Design review of the part built by this model. Coordinates are the model's own, in mm. Face numbers are marked on the shaded views. A direction names the side the tool comes from. Give positions to 0.01 mm unless a question says otherwise; leave off trailing zeros. Loops run counter-clockwise (first coordinate to the right, second up) from the corner with the lowest first, then second, coordinate; pieces in that order, holes last. Notation, with made-up numbers: M 62.5,27 L 76.5,27 A17 cw 76.5,55 Z; hole C 36,43.25 d4. An arc over 180 degrees is marked long. Use a Markdown table: item, result. Add a question column.
(1) Insertion check: pin 1 Ø10 at (x, z) = (-5, -10.5) entering from -Y; pin 2 Ø3 at (x, z) = (-13, 1) entering from +Y; pin 3 Ø0.9 at (x, y) = (32.5, -0.5) entering from -Z. Each pin has a flat end and moves straight along its axis. Give the tip position at first contact, or say it passes through.
(2) For probe 1 along Y at (x, z) = (0, 3.9); probe 2 along Y at (x, z) = (0, -8); probe 3 along X at (y, z) = (-32.5, -7.75), list the stretches that pass through material, from the lowest coordinate up.
(3) For the marked faces 1 and 2, list the 3-axis set-ups (+Z, -Z, +X, -X, +Y, -Y) from which the entire face can be reached by the end or side of a thin tool; tool diameter is ignored.
(4) Add section D-D, the plane z = 3.5. Give the boundary of the cut face in (x, y).
(5) Add section B-B, the plane y = -32.5. Give the boundary of the cut face in (x, z).
(6) Add section A-A, the plane z = -10.75. Give the boundary of the cut face in (x, y), then the cut area to 3 significant figures.
(7) Draft analysis for pull direction X (two halves, no side actions). For the marked faces 3 and 4, state which applies: pulls with the +X half, pulls with the -X half, needs draft (parallel to the pull), parting line crosses it, or undercut.
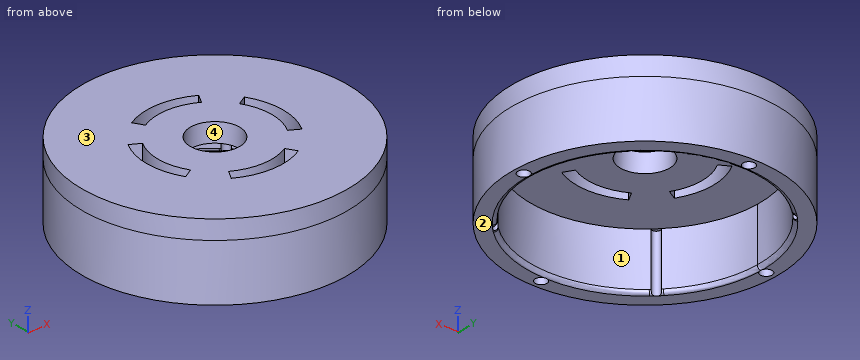
```python
from build123d import *

# Parameters (mm, degrees)
SKETCH_2_R          = 35
SKETCH_2_R_2        = 6.5
EXTRUDE_1_DEPTH     = 5
EXTRUDE_START       = 15
SKETCH_3_R          = 35
SKETCH_3_R_2        = 30.1
EXTRUDE_2_DEPTH     = 15
SKETCH_4_R          = 1.55
CUT_EXTRUDE_1_DEPTH = 10
CUT_EXTRUDE_2_DEPTH = 52.720402164
CUT_EXTRUDE_5_DEPTH = 15
FILLET_1_R          = 1


with BuildPart() as part:
    # 草图2 → 凸台-拉伸1 (new body)
    with BuildSketch(Plane.XY):
        Circle(SKETCH_2_R)
        Circle(SKETCH_2_R_2, mode=Mode.SUBTRACT)
    extrude(amount=EXTRUDE_1_DEPTH)

    # 草图3 → 凸台-拉伸2 (add)
    with BuildSketch(Plane(origin=(0, 0, 0), x_dir=(-1, 0, 0), z_dir=(0, 0, -1)).offset(EXTRUDE_START)):
        Circle(SKETCH_3_R)
        Circle(SKETCH_3_R_2, mode=Mode.SUBTRACT)
    extrude(amount=-EXTRUDE_2_DEPTH)

    # 草图4 → 切除-拉伸1 (cut)
    with BuildSketch(Plane(origin=(0, 0, -15), x_dir=(-1, 0, 0), z_dir=(0, 0, -1))):
        with Locations((0, 32.5)):
            Circle(SKETCH_4_R)
        with Locations((32.5, 0)):
            Circle(SKETCH_4_R)
        with Locations((0, -32.5)):
            Circle(SKETCH_4_R)
        with Locations((-32.5, 0)):
            Circle(SKETCH_4_R)
    extrude(amount=-CUT_EXTRUDE_1_DEPTH, mode=Mode.SUBTRACT)

    # 草图5 → 切除-拉伸2 (cut, through all)
    with BuildSketch(Plane(origin=(0, 0, 0), x_dir=(-1, 0, 0), z_dir=(0, 0, -1))):
        with BuildLine():
            Line((12.990381057, -7.5), (15.588457268, -9))
            ThreePointArc((15.588457268, -9), (18, 0), (15.588457268, 9))
            Line((15.588457268, 9), (12.990381057, 7.5))
            ThreePointArc((12.990381057, 7.5), (15, 0), (12.990381057, -7.5))
        make_face()
        with BuildLine():
            Line((-7.5, 12.990381057), (-9, 15.588457268))
            ThreePointArc((-9, 15.588457268), (0, 18), (9, 15.588457268))
            Line((9, 15.588457268), (7.5, 12.990381057))
            ThreePointArc((7.5, 12.990381057), (0, 15), (-7.5, 12.990381057))
        make_face()
        with BuildLine():
            Line((-7.5, -12.990381057), (-9, -15.588457268))
            ThreePointArc((-9, -15.588457268), (0, -18), (9, -15.588457268))
            Line((9, -15.588457268), (7.5, -12.990381057))
            ThreePointArc((7.5, -12.990381057), (0, -15), (-7.5, -12.990381057))
        make_face()
        with BuildLine():
            Line((-12.990381057, 7.5), (-15.588457268, 9))
            ThreePointArc((-15.588457268, 9), (-18, 0), (-15.588457268, -9))
            Line((-15.588457268, -9), (-12.990381057, -7.5))
            ThreePointArc((-12.990381057, -7.5), (-15, 0), (-12.990381057, 7.5))
        make_face()
    extrude(amount=-CUT_EXTRUDE_2_DEPTH, mode=Mode.SUBTRACT)

    # 草图9 → 切除-拉伸5 (cut)
    with BuildSketch(Plane(origin=(0, 0, -15), x_dir=(-1, 0, 0), z_dir=(0, 0, -1))):
        with BuildLine():
            ThreePointArc((-22.013313369, 20.528615017), (-22.026376234, 22.026376234), (-20.528615017, 22.013313369))
            ThreePointArc((-20.528615017, 22.013313369), (-21.283914114, 21.283914114), (-22.013313369, 20.528615017))
        make_face()
        with BuildLine():
            ThreePointArc((20.528615017, 22.013313369), (22.026376234, 22.026376234), (22.013313369, 20.528615017))
            ThreePointArc((22.013313369, 20.528615017), (21.283914114, 21.283914114), (20.528615017, 22.013313369))
        make_face()
        with BuildLine():
            ThreePointArc((22.013313369, -20.528615017), (22.026376234, -22.026376234), (20.528615017, -22.013313369))
            ThreePointArc((20.528615017, -22.013313369), (21.283914114, -21.283914114), (22.013313369, -20.528615017))
        make_face()
        with BuildLine():
            ThreePointArc((-20.528615017, -22.013313369), (-22.026376234, -22.026376234), (-22.013313369, -20.528615017))
            ThreePointArc((-22.013313369, -20.528615017), (-21.283914114, -21.283914114), (-20.528615017, -22.013313369))
        make_face()
    extrude(amount=-CUT_EXTRUDE_5_DEPTH, mode=Mode.SUBTRACT)

    # 圆角1
    # the kernel refuses this fillet: 1 mm, written as the material it takes off along each edge
    with BuildSketch(Plane(origin=(0, 0, -15), x_dir=(-0.7403558797037455, 0.6722151228498904, 0), z_dir=(-0.6722151228498904, -0.7403558797037455, 0))) as fillet_1_piece_1:
        with BuildLine():
            CenterArc((30.1 + FILLET_1_R, -FILLET_1_R), FILLET_1_R, 90, 90)
            Line((30.1, -FILLET_1_R), (30.1, 0))
            Line((30.1, 0), (30.1 + FILLET_1_R, 0))
        make_face()
    revolve(axis=Axis((0, 0, -15), (0, 0, -1)), revolution_arc=95.523479776, mode=Mode.SUBTRACT)
    with BuildSketch(Plane(origin=(0, 0, -15), x_dir=(0.6722151228498918, 0.7403558797037441, 0), z_dir=(-0.7403558797037441, 0.6722151228498918, 0))) as fillet_1_piece_2:
        with BuildLine():
            CenterArc((30.1 + FILLET_1_R, -FILLET_1_R), FILLET_1_R, 90, 90)
            Line((30.1, -FILLET_1_R), (30.1, 0))
            Line((30.1, 0), (30.1 + FILLET_1_R, 0))
        make_face()
    revolve(axis=Axis((0, 0, -15), (0, 0, -1)), revolution_arc=95.523479776, mode=Mode.SUBTRACT)
    with BuildSketch(Plane(origin=(0, 0, -15), x_dir=(0.7403558797037453, -0.6722151228498905, 0), z_dir=(0.6722151228498905, 0.7403558797037453, 0))) as fillet_1_piece_3:
        with BuildLine():
            CenterArc((30.1 + FILLET_1_R, -FILLET_1_R), FILLET_1_R, 90, 90)
            Line((30.1, -FILLET_1_R), (30.1, 0))
            Line((30.1, 0), (30.1 + FILLET_1_R, 0))
        make_face()
    revolve(axis=Axis((0, 0, -15), (0, 0, -1)), revolution_arc=95.523479776, mode=Mode.SUBTRACT)
    with BuildSketch(Plane(origin=(0, 0, -15), x_dir=(-1, 0, 0), z_dir=(0, -1, 0))) as fillet_1_piece_4:
        with BuildLine():
            CenterArc((30.1 + FILLET_1_R, -FILLET_1_R), FILLET_1_R, 90, 90)
            Line((30.1, -FILLET_1_R), (30.1, 0))
            Line((30.1, 0), (30.1 + FILLET_1_R, 0))
        make_face()
    revolve(axis=Axis((0, 0, -15), (0, 0, -1)), revolution_arc=47.760430641, mode=Mode.SUBTRACT)
    with BuildSketch(Plane(origin=(0, 0, -15), x_dir=(-0.6722320403041436, -0.7403405189428228, 0), z_dir=(0.7403405189428228, -0.6722320403041436, 0))) as fillet_1_piece_5:
        with BuildLine():
            CenterArc((30.1 + FILLET_1_R, -FILLET_1_R), FILLET_1_R, 90, 90)
            Line((30.1, -FILLET_1_R), (30.1, 0))
            Line((30.1, 0), (30.1 + FILLET_1_R, 0))
        make_face()
    revolve(axis=Axis((0, 0, -15), (0, 0, -1)), revolution_arc=47.760430641, mode=Mode.SUBTRACT)


solid = part.part
```
Established:
| question | item | result |
|---|---|---|
| 1 | pin 1 | y = -35 |
| 1 | pin 2 | y = 33.06 |
| 1 | pin 3 | z = -5 |
| 2 | probe 1 | -35 to -18, -15 to -6.5, 6.5 to 15, 18 to 35 |
| 2 | probe 2 | -35 to -34.05, -30.95 to -30.1, 30.1 to 30.95, 34.05 to 35 |
| 2 | probe 3 | -12.99 to -1.55, 1.55 to 12.99 |
| 3 | face 1 | -Z |
| 3 | face 2 | -Z, +X, -X, +Y, -Y |
| 4 | outline | C 0,0 d70; hole M -15.59,-9 L -12.99,-7.5 A15 cw -12.99,7.5 L -15.59,9 A18 ccw Z; hole M -9,-15.59 A18 ccw 9,-15.59 L 7.5,-12.99 A15 cw -7.5,-12.99 Z; hole M -9,15.59 L -7.5,12.99 A15 cw 7.5,12.99 L 9,15.59 A18 ccw Z; hole C 0,0 d13; hole M 12.99,-7.5 L 15.59,-9 A18 ccw 15.59,9 L 12.99,7.5 A15 cw Z |
| 5 | outline | M -12.99,-15 L -1.55,-15 L -1.55,-5 L 1.55,-5 L 1.55,-15 L 12.99,-15 L 12.99,5 L -12.99,5 Z |
| 6 | outline | C 0,0 d70; hole C -32.5,0 d3.1; hole M -22.01,-20.53 A1.05 ccw long -20.53,-22.01 A30.1 ccw 20.53,-22.01 A1.05 ccw long 22.01,-20.53 A30.1 ccw 22.01,20.53 A1.05 ccw long 20.53,22.01 A30.1 ccw -20.53,22.01 A1.05 ccw long -22.01,20.53 A30.1 ccw Z; hole C 0,-32.5 d3.1; hole C 0,32.5 d3.1; hole C 32.5,0 d3.1 |
| 6 | area | 965 mm^2 |
| 7 | face 3 | needs draft |
| 7 | face 4 | undercut |
